```python
from build123d import *

# Parameters (mm, degrees)
SKETCH_1_W                  = 186
SKETCH_1_H                  = 60
EXTRUDE_1_DEPTH             = 3
SKETCH_2_W                  = 3
SKETCH_2_H                  = 60
EXTRUDE_2_DEPTH             = 40
SKETCH_3_W                  = 60
SKETCH_3_H                  = 3
EXTRUDE_3_DEPTH             = 20
SKETCH_4_R                  = 1.75
CUT_EXTRUDE_1_DEPTH         = 124.567795157
PATTERN_LINEAR_1_COUNT      = 3
PATTERN_LINEAR_1_PITCH      = 20
PATTERN_LINEAR_1_COUNT_DIR2 = 2
PATTERN_LINEAR_1_PITCH_DIR2 = 10
MIRROR_4_COPY_1_SKETCH_R    = 1.75
MIRROR_4_COPY_1_DEPTH       = 124.567795157
MIRROR_4_COPY_2_SKETCH_R    = 1.75
MIRROR_4_COPY_2_DEPTH       = 124.567795157
MIRROR_4_COPY_3_SKETCH_R    = 1.75
MIRROR_4_COPY_3_DEPTH       = 124.567795157
MIRROR_4_COPY_4_SKETCH_R    = 1.75
MIRROR_4_COPY_4_DEPTH       = 124.567795157
MIRROR_4_COPY_5_SKETCH_R    = 1.75
MIRROR_4_COPY_5_DEPTH       = 124.567795157
SKETCH_5_R                  = 1
CUT_EXTRUDE_2_DEPTH         = 3
SKETCH_6_R                  = 1
CUT_EXTRUDE_3_DEPTH         = 3
SKETCH_7_R                  = 1
CUT_EXTRUDE_4_DEPTH         = 3
PATTERN_LINEAR_2_COUNT      = 3
PATTERN_LINEAR_2_PITCH      = 20
PATTERN_LINEAR_2_COUNT_DIR2 = 2
PATTERN_LINEAR_2_PITCH_DIR2 = 10
MIRROR_6_COPY_1_SKETCH_R    = 1
MIRROR_6_COPY_1_DEPTH       = 3
MIRROR_6_COPY_2_SKETCH_R    = 1
MIRROR_6_COPY_2_DEPTH       = 3
MIRROR_6_COPY_3_SKETCH_R    = 1
MIRROR_6_COPY_3_DEPTH       = 3
MIRROR_6_COPY_4_SKETCH_R    = 1
MIRROR_6_COPY_4_DEPTH       = 3
MIRROR_6_COPY_5_SKETCH_R    = 1
MIRROR_6_COPY_5_DEPTH       = 3
HOLE_WIZARD_M3_1_D          = 2.5
HOLE_WIZARD_M3_2_D          = 2.5
SKETCH_12_R                 = 15
CUT_EXTRUDE_5_DEPTH         = 124.567795157
FILLET_2_R                  = 2
FILLET_3_R                  = 2
FILLET_4_R                  = 2
FILLET_5_R                  = 3


with BuildPart() as part:
    # 草图1 → 凸台-拉伸1 (new body)
    with BuildSketch(Plane(origin=(0, 0, 0), x_dir=(1, 0, 0), z_dir=(0, 1, 0))):
        Rectangle(SKETCH_1_W, SKETCH_1_H)
    extrude(amount=EXTRUDE_1_DEPTH)

    # 草图2 → 凸台-拉伸2 (add)
    with BuildSketch(Plane.XZ):
        with Locations((-91.5, 0)):
            Rectangle(SKETCH_2_W, SKETCH_2_H)
    extrude_2 = extrude(amount=EXTRUDE_2_DEPTH)

    # 草图3 → 凸台-拉伸3 (add)
    with BuildSketch(Plane.ZY.offset(93)):
        with Locations((0, -38.5)):
            Rectangle(SKETCH_3_W, SKETCH_3_H)
    extrude_3 = extrude(amount=EXTRUDE_3_DEPTH)

    # 草图4 → 切除-拉伸1 (cut, through all)
    with BuildSketch(Plane(origin=(0, -37, 0), x_dir=(1, 0, 0), z_dir=(0, 1, 0))):
        with Locations(Location((-98, -20, 0), (0, 0, 270))):
            Circle(SKETCH_4_R)
    cut_extrude_1 = extrude(amount=-CUT_EXTRUDE_1_DEPTH, mode=Mode.SUBTRACT)

    # 阵列(线性)1: Cut-Extrude 1 3 × 2
    with Locations(*[(-j * PATTERN_LINEAR_1_PITCH_DIR2, 0, -i * PATTERN_LINEAR_1_PITCH) for i in range(PATTERN_LINEAR_1_COUNT) for j in range(PATTERN_LINEAR_1_COUNT_DIR2) if (i, j) != (0, 0)]):
        add(cut_extrude_1, mode=Mode.SUBTRACT)

    # 镜向4: 凸台-拉伸2, 凸台-拉伸3, 切除-拉伸1 across plane
    add(extrude_2.mirror(Plane(origin=(0, 0, 0), x_dir=(0, 0, 1), z_dir=(1, 0, 0))))
    add(extrude_3.mirror(Plane(origin=(0, 0, 0), x_dir=(0, 0, 1), z_dir=(1, 0, 0))))
    add(cut_extrude_1.mirror(Plane(origin=(0, 0, 0), x_dir=(0, 0, 1), z_dir=(1, 0, 0))), mode=Mode.SUBTRACT)

    # 镜向4 copy 1 sketch → 镜向4 copy 1 (cut, through all)
    with BuildSketch(Plane(origin=(10, -37, 0), x_dir=(-1, 0, 0), z_dir=(0, 1, 0))):
        with Locations((-98, 20)):
            Circle(MIRROR_4_COPY_1_SKETCH_R)
    extrude(amount=-MIRROR_4_COPY_1_DEPTH, mode=Mode.SUBTRACT)

    # 镜向4 copy 2 sketch → 镜向4 copy 2 (cut, through all)
    with BuildSketch(Plane(origin=(0, -37, -20), x_dir=(-1, 0, 0), z_dir=(0, 1, 0))):
        with Locations((-98, 20)):
            Circle(MIRROR_4_COPY_2_SKETCH_R)
    extrude(amount=-MIRROR_4_COPY_2_DEPTH, mode=Mode.SUBTRACT)

    # 镜向4 copy 3 sketch → 镜向4 copy 3 (cut, through all)
    with BuildSketch(Plane(origin=(10, -37, -20), x_dir=(-1, 0, 0), z_dir=(0, 1, 0))):
        with Locations((-98, 20)):
            Circle(MIRROR_4_COPY_3_SKETCH_R)
    extrude(amount=-MIRROR_4_COPY_3_DEPTH, mode=Mode.SUBTRACT)

    # 镜向4 copy 4 sketch → 镜向4 copy 4 (cut, through all)
    with BuildSketch(Plane(origin=(0, -37, -40), x_dir=(-1, 0, 0), z_dir=(0, 1, 0))):
        with Locations((-98, 20)):
            Circle(MIRROR_4_COPY_4_SKETCH_R)
    extrude(amount=-MIRROR_4_COPY_4_DEPTH, mode=Mode.SUBTRACT)

    # 镜向4 copy 5 sketch → 镜向4 copy 5 (cut, through all)
    with BuildSketch(Plane(origin=(10, -37, -40), x_dir=(-1, 0, 0), z_dir=(0, 1, 0))):
        with Locations((-98, 20)):
            Circle(MIRROR_4_COPY_5_SKETCH_R)
    extrude(amount=-MIRROR_4_COPY_5_DEPTH, mode=Mode.SUBTRACT)

    # 草图5 → 切除-拉伸2 (cut)
    with BuildSketch(Plane(origin=(0, 3, 0), x_dir=(1, 0, 0), z_dir=(0, 1, 0))):
        with Locations(Location((0, -26, 0), (0, 0, 270))):
            Circle(SKETCH_5_R)
    extrude(amount=-CUT_EXTRUDE_2_DEPTH, mode=Mode.SUBTRACT)

    # 草图6 → 切除-拉伸3 (cut)
    with BuildSketch(Plane(origin=(0, 3, 0), x_dir=(1, 0, 0), z_dir=(0, 1, 0))):
        with Locations(Location((-17.45, 24.5, 0), (0, 0, 270))):
            Circle(SKETCH_6_R)
    cut_extrude_3 = extrude(amount=-CUT_EXTRUDE_3_DEPTH, mode=Mode.SUBTRACT)

    # 镜向5: 切除-拉伸3 across plane
    add(cut_extrude_3.mirror(Plane(origin=(0, 0, 0), x_dir=(0, 0, 1), z_dir=(1, 0, 0))), mode=Mode.SUBTRACT)

    # 草图7 → 切除-拉伸4 (cut)
    with BuildSketch(Plane(origin=(0, 3, 0), x_dir=(1, 0, 0), z_dir=(0, 1, 0))):
        with Locations(Location((-70, -20, 0), (0, 0, 270))):
            Circle(SKETCH_7_R)
    cut_extrude_4 = extrude(amount=-CUT_EXTRUDE_4_DEPTH, mode=Mode.SUBTRACT)

    # 阵列(线性)2: Cut-Extrude 4 3 × 2
    with Locations(*[(-j * PATTERN_LINEAR_2_PITCH_DIR2, 0, -i * PATTERN_LINEAR_2_PITCH) for i in range(PATTERN_LINEAR_2_COUNT) for j in range(PATTERN_LINEAR_2_COUNT_DIR2) if (i, j) != (0, 0)]):
        add(cut_extrude_4, mode=Mode.SUBTRACT)

    # 镜向6: 切除-拉伸4 across plane
    add(cut_extrude_4.mirror(Plane(origin=(0, 0, 0), x_dir=(0, 0, 1), z_dir=(1, 0, 0))), mode=Mode.SUBTRACT)

    # 镜向6 copy 1 sketch → 镜向6 copy 1 (cut)
    with BuildSketch(Plane(origin=(10, 3, 0), x_dir=(-1, 0, 0), z_dir=(0, 1, 0))):
        with Locations((-70, 20)):
            Circle(MIRROR_6_COPY_1_SKETCH_R)
    extrude(amount=-MIRROR_6_COPY_1_DEPTH, mode=Mode.SUBTRACT)

    # 镜向6 copy 2 sketch → 镜向6 copy 2 (cut)
    with BuildSketch(Plane(origin=(0, 3, -20), x_dir=(-1, 0, 0), z_dir=(0, 1, 0))):
        with Locations((-70, 20)):
            Circle(MIRROR_6_COPY_2_SKETCH_R)
    extrude(amount=-MIRROR_6_COPY_2_DEPTH, mode=Mode.SUBTRACT)

    # 镜向6 copy 3 sketch → 镜向6 copy 3 (cut)
    with BuildSketch(Plane(origin=(10, 3, -20), x_dir=(-1, 0, 0), z_dir=(0, 1, 0))):
        with Locations((-70, 20)):
            Circle(MIRROR_6_COPY_3_SKETCH_R)
    extrude(amount=-MIRROR_6_COPY_3_DEPTH, mode=Mode.SUBTRACT)

    # 镜向6 copy 4 sketch → 镜向6 copy 4 (cut)
    with BuildSketch(Plane(origin=(0, 3, -40), x_dir=(-1, 0, 0), z_dir=(0, 1, 0))):
        with Locations((-70, 20)):
            Circle(MIRROR_6_COPY_4_SKETCH_R)
    extrude(amount=-MIRROR_6_COPY_4_DEPTH, mode=Mode.SUBTRACT)

    # 镜向6 copy 5 sketch → 镜向6 copy 5 (cut)
    with BuildSketch(Plane(origin=(10, 3, -40), x_dir=(-1, 0, 0), z_dir=(0, 1, 0))):
        with Locations((-70, 20)):
            Circle(MIRROR_6_COPY_5_SKETCH_R)
    extrude(amount=-MIRROR_6_COPY_5_DEPTH, mode=Mode.SUBTRACT)

    # M3 螺纹孔1 (through all)
    with Locations(Plane(origin=(0, 3, 0), x_dir=(1, 0, 0), z_dir=(0, 1, 0))):
        with Locations((-80, -20), (-70, -20), (-70, 0), (-80, 0), (-70, 20), (-80, 20), (70, -20), (80, -20), (70, 0), (80, 0), (70, 20), (80, 20)):
            Hole(HOLE_WIZARD_M3_1_D / 2)

    # M3 螺纹孔2 (through all)
    with Locations(Plane(origin=(0, 3, 0), x_dir=(1, 0, 0), z_dir=(0, 1, 0))):
        with Locations((-17.45, 24.5), (17.45, 24.5), (0, -26)):
            Hole(HOLE_WIZARD_M3_2_D / 2)

    # 草图12 → 切除-拉伸5 (cut, through all)
    with BuildSketch(Plane(origin=(0, -37, 0), x_dir=(1, 0, 0), z_dir=(0, 1, 0))):
        with Locations((-120, 0)):
            Circle(SKETCH_12_R)
    cut_extrude_5 = extrude(amount=-CUT_EXTRUDE_5_DEPTH, mode=Mode.SUBTRACT)

    # 镜向7: 切除-拉伸5 across plane
    add(cut_extrude_5.mirror(Plane(origin=(0, 0, 0), x_dir=(0, 0, 1), z_dir=(1, 0, 0))), mode=Mode.SUBTRACT)

    # 圆角2
    fillet_2_edges = [part.edges().sort_by_distance(p)[0] for p in [
        (-90, 0, 0),
        (-93, 3, 0),
    ]]
    fillet(fillet_2_edges, radius=FILLET_2_R)

    # 圆角3
    fillet_3_edges = [part.edges().sort_by_distance(p)[0] for p in [
        (93, 3, 0),
        (90, 0, 0),
    ]]
    fillet(fillet_3_edges, radius=FILLET_3_R)

    # 圆角4
    fillet_4_edges = [part.edges().sort_by_distance(p)[0] for p in [
        (-90, -40, 0),
        (-93, -37, 0),
        (90, -40, 0),
        (93, -37, 0),
    ]]
    fillet(fillet_4_edges, radius=FILLET_4_R)

    # 圆角5
    fillet_5_edges = [part.edges().sort_by_distance(p)[0] for p in [
        (-113, -38.5, -30),
        (-113, -38.5, 30),
        (113, -38.5, 30),
        (113, -38.5, -30),
    ]]
    fillet(fillet_5_edges, radius=FILLET_5_R)


solid = part.part
```
Check sheet for the modelled part. Datum: model origin and axes. Units: mm. A direction names the side the tool comes from. Round coordinates to 2 decimals unless told otherwise and drop trailing zeros. Order: outer loops, then holes, each group sorted by start corner. A loop starts at its lowest first (then second) coordinate and runs counter-clockwise, first axis right, second up. Notation, with made-up numbers: (64, 80) - (88, 80) arc R6 cw to (88, 84) - close; hole circle Ø4 at (21.5, 18.25). An arc over 180 degrees is marked (long way). Write item = value, one per line.
Q1. Thickness scan on line 1 along Z through (x, y) = (-98, -39.05); line 2 along X through (y, z) = (-4.5, 15); line 3 along Y through (x, z) = (77, -18). Record the ranges inside material, lowest first.
Computed:
line_1 = -30 to -21.75, -18.25 to -1.75, 1.75 to 18.25, 21.75 to 30
line_2 = -93 to -90, 90 to 93
line_3 = 0 to 3
Q2. Draft check along Z on faces 1 (the face through (90, -20, 0)), 2 (the face through (-105, -38, 0)), 3 (the face through (-25, 1, 30)), 4 (the face through (-25, 1, -30)). Enter one of: pulls with the +Z half, pulls with the -Z half, needs draft (parallel to the pull), parting line crosses it, or undercut.
Computed:
face_1 = needs draft
face_2 = undercut
face_3 = pulls with the +Z half
face_4 = pulls with the -Z half
Q3. Section check A-A (y = -21). Record the boundary of the cut face in (x, z).
Computed:
outline = (-93, -30) - (-90, -30) - (-90, 30) - (-93, 30) - close; (90, -30) - (93, -30) - (93, 30) - (90, 30) - close
Q4. Tool access check on faces 5 (the face through (-104, -37, 0)), 6 (the face through (-1, 0, 0)), 7 (the face through (105, -38, 0)), 8 (the face through (104, -37, 0)). Record the directions out of +Z, -Z, +X, -X, +Y, -Y that give a thin tool (end or side, any length) a straight path to the whole face; none if there is none.
Computed:
face_5 = +Z, -Z, -X, +Y
face_6 = +Z, -Z, -Y
face_7 = +X, +Y, -Y
face_8 = +Z, -Z, +X, +Y
Q5. Section check C-C (x = -22). Record the boundary of the cut face in (y, z), and give its area (3 significant figures).
Computed:
outline = (0, -30) - (3, -30) - (3, 30) - (0, 30) - close
area = 180 mm^2
Q6. Section check B-B (z = 9). Record the boundary of the cut face in (x, y).
Computed:
outline = (-108, -40) - (-92, -40) arc R2 ccw to (-90, -38) - (-90, -2) arc R2 cw to (-88, 0) - (88, 0) arc R2 cw to (90, -2) - (90, -38) arc R2 ccw to (92, -40) - (108, -40) - (108, -37) - (95, -37) arc R2 cw to (93, -35) - (93, 1) arc R2 ccw to (91, 3) - (-91, 3) arc R2 ccw to (-93, 1) - (-93, -35) arc R2 cw to (-95, -37) - (-108, -37) - close
Q7. Go/stop test with flat-tipped pins: pin 1 (4 mm diameter, centred on x = 37.5, z = 12, fed in from -Y); pin 2 (12 mm diameter, centred on y = -23, z = 20, fed in from -X); pin 3 (5.5 mm diameter, centred on x = 108.5, z = 14.5, fed in from +Y). Record where each tip stops, or that it passes through.
Computed:
pin_1 = 0
pin_2 = -93
pin_3 = -37
